from build123d import *

# Parameters (mm, degrees)
F0_R     = 8
F0_W     = 6.01
F0_H     = 18.1
F1_DEPTH = 6


with BuildPart() as f1:
    # F0 (on Front) → F1 (new body)
    with BuildSketch(Plane.XZ):
        Polygon((133.745999, -172.696896), (-31.254001, -172.696896), (-31.254001, -207.736896), (-25.244001, -207.736896), (-25.244001, -225.836896), (-31.254001, -225.836896), (-31.254001, -275.836896), (-25.244001, -275.836896), (-25.244001, -293.936896), (-31.254001, -293.936896), (-31.254001, -316.696896), (26.745999, -316.696896), (26.745999, -310.686896), (44.845999, -310.686896), (44.845999, -316.696896), (88.745999, -316.696896), (88.745999, -310.686896), (106.845999, -310.686896), (106.845999, -316.696896), (730.645999, -316.696896), (730.645999, -310.686896), (748.745999, -310.686896), (748.745999, -316.696896), (792.645999, -316.696896), (792.645999, -310.686896), (810.745999, -310.686896), (810.745999, -316.696896), (862.745999, -316.696896), (862.745999, -293.926896), (868.545999, -293.926896), (868.545999, -291.926896), (865.745999, -289.926896), (865.745999, -279.926896), (868.545999, -277.926896), (868.545999, -275.926896), (862.745999, -275.926896), (862.745999, -225.906896), (868.545999, -225.906896), (868.545999, -223.906896), (865.745999, -221.906896), (865.745999, -211.906896), (868.545999, -209.906896), (868.545999, -207.906896), (862.745999, -207.906896), (862.745999, -172.696896), (691.745999, -172.696896), (691.745999, -166.896896), (689.745999, -166.896896), (687.745999, -169.696896), (677.745999, -169.696896), (675.745999, -166.896896), (673.745999, -166.896896), (673.745999, -172.696896), (511.745999, -172.696896), (511.745999, -166.896896), (509.745999, -166.896896), (507.745999, -169.696896), (497.745999, -169.696896), (495.745999, -166.896896), (493.745999, -166.896896), (493.745999, -172.696896), (331.745999, -172.696896), (331.745999, -166.896896), (329.745999, -166.896896), (327.745999, -169.696896), (317.745999, -169.696896), (315.745999, -166.896896), (313.745999, -166.896896), (313.745999, -172.696896), (151.745999, -172.696896), (151.745999, -166.736896), (149.745999, -166.736896), (147.745999, -169.696896), (137.745999, -169.696896), (135.745999, -166.736896), (133.745999, -166.736896), align=None)
        with Locations((-6.254001, -291.696896)):
            Circle(F0_R, mode=Mode.SUBTRACT)
        with Locations((44.373021, -291.696896)):
            Circle(F0_R, mode=Mode.SUBTRACT)
        with Locations((94.373021, -291.696896)):
            Circle(F0_R, mode=Mode.SUBTRACT)
        with Locations((144.373021, -291.696896)):
            Circle(F0_R, mode=Mode.SUBTRACT)
        with Locations((161.750999, -284.886896)):
            Rectangle(F0_W, F0_H, mode=Mode.SUBTRACT)
        with Locations((194.373021, -291.696896)):
            Circle(F0_R, mode=Mode.SUBTRACT)
        with Locations((244.373021, -291.696896)):
            Circle(F0_R, mode=Mode.SUBTRACT)
        with Locations((294.373021, -291.696896)):
            Circle(F0_R, mode=Mode.SUBTRACT)
        with Locations((344.373021, -291.696896)):
            Circle(F0_R, mode=Mode.SUBTRACT)
        with Locations((394.373021, -291.696896)):
            Circle(F0_R, mode=Mode.SUBTRACT)
        with Locations((326.950999, -284.886896)):
            Rectangle(F0_W, F0_H, mode=Mode.SUBTRACT)
        with Locations((444.373021, -291.696896)):
            Circle(F0_R, mode=Mode.SUBTRACT)
        with Locations((494.373021, -291.696896)):
            Circle(F0_R, mode=Mode.SUBTRACT)
        with Locations((510.540999, -284.886896)):
            Rectangle(F0_W, F0_H, mode=Mode.SUBTRACT)
        with Locations((544.373021, -291.696896)):
            Circle(F0_R, mode=Mode.SUBTRACT)
        with Locations((594.373021, -291.696896)):
            Circle(F0_R, mode=Mode.SUBTRACT)
        with Locations((644.373021, -291.696896)):
            Circle(F0_R, mode=Mode.SUBTRACT)
        with Locations((694.373021, -291.696896)):
            Circle(F0_R, mode=Mode.SUBTRACT)
        with Locations((744.373021, -291.696896)):
            Circle(F0_R, mode=Mode.SUBTRACT)
        with Locations((675.740999, -284.886896)):
            Rectangle(F0_W, F0_H, mode=Mode.SUBTRACT)
        with Locations((794.373021, -291.696896)):
            Circle(F0_R, mode=Mode.SUBTRACT)
        with Locations((844.373021, -291.696896)):
            Circle(F0_R, mode=Mode.SUBTRACT)
        with Locations((-6.254001, -241.696896)):
            Circle(F0_R, mode=Mode.SUBTRACT)
        with Locations((44.373021, -241.696896)):
            Circle(F0_R, mode=Mode.SUBTRACT)
        with Locations((94.373021, -241.696896)):
            Circle(F0_R, mode=Mode.SUBTRACT)
        with Locations((144.373021, -241.696896)):
            Circle(F0_R, mode=Mode.SUBTRACT)
        with Locations((161.750999, -216.946896)):
            Rectangle(F0_W, F0_H, mode=Mode.SUBTRACT)
        with Locations((194.373021, -241.696896)):
            Circle(F0_R, mode=Mode.SUBTRACT)
        with Locations((244.373021, -241.696896)):
            Circle(F0_R, mode=Mode.SUBTRACT)
        with Locations((294.373021, -241.696896)):
            Circle(F0_R, mode=Mode.SUBTRACT)
        with Locations((344.373021, -241.696896)):
            Circle(F0_R, mode=Mode.SUBTRACT)
        with Locations((394.373021, -241.696896)):
            Circle(F0_R, mode=Mode.SUBTRACT)
        with Locations((326.950999, -216.946896)):
            Rectangle(F0_W, F0_H, mode=Mode.SUBTRACT)
        with Locations((-6.254001, -191.696896)):
            Circle(F0_R, mode=Mode.SUBTRACT)
        with Locations((44.373021, -191.696896)):
            Circle(F0_R, mode=Mode.SUBTRACT)
        with Locations((94.373021, -191.696896)):
            Circle(F0_R, mode=Mode.SUBTRACT)
        with Locations((144.373021, -191.696896)):
            Circle(F0_R, mode=Mode.SUBTRACT)
        with Locations((194.373021, -191.696896)):
            Circle(F0_R, mode=Mode.SUBTRACT)
        with Locations((244.373021, -191.696896)):
            Circle(F0_R, mode=Mode.SUBTRACT)
        with Locations((294.373021, -191.696896)):
            Circle(F0_R, mode=Mode.SUBTRACT)
        with Locations((344.373021, -191.696896)):
            Circle(F0_R, mode=Mode.SUBTRACT)
        with Locations((394.373021, -191.696896)):
            Circle(F0_R, mode=Mode.SUBTRACT)
        with Locations((444.373021, -241.696896)):
            Circle(F0_R, mode=Mode.SUBTRACT)
        with Locations((494.373021, -241.696896)):
            Circle(F0_R, mode=Mode.SUBTRACT)
        with Locations((544.373021, -241.696896)):
            Circle(F0_R, mode=Mode.SUBTRACT)
        with Locations((594.373021, -241.696896)):
            Circle(F0_R, mode=Mode.SUBTRACT)
        with Locations((510.540999, -216.946896)):
            Rectangle(F0_W, F0_H, mode=Mode.SUBTRACT)
        with Locations((644.373021, -241.696896)):
            Circle(F0_R, mode=Mode.SUBTRACT)
        with Locations((694.373021, -241.696896)):
            Circle(F0_R, mode=Mode.SUBTRACT)
        with Locations((744.373021, -241.696896)):
            Circle(F0_R, mode=Mode.SUBTRACT)
        with Locations((794.373021, -241.696896)):
            Circle(F0_R, mode=Mode.SUBTRACT)
        with Locations((844.373021, -241.696896)):
            Circle(F0_R, mode=Mode.SUBTRACT)
        with Locations((675.740999, -216.946896)):
            Rectangle(F0_W, F0_H, mode=Mode.SUBTRACT)
        with Locations((444.373021, -191.696896)):
            Circle(F0_R, mode=Mode.SUBTRACT)
        with Locations((494.373021, -191.696896)):
            Circle(F0_R, mode=Mode.SUBTRACT)
        with Locations((544.373021, -191.696896)):
            Circle(F0_R, mode=Mode.SUBTRACT)
        with Locations((594.373021, -191.696896)):
            Circle(F0_R, mode=Mode.SUBTRACT)
        with Locations((644.373021, -191.696896)):
            Circle(F0_R, mode=Mode.SUBTRACT)
        with Locations((694.373021, -191.696896)):
            Circle(F0_R, mode=Mode.SUBTRACT)
        with Locations((744.373021, -191.696896)):
            Circle(F0_R, mode=Mode.SUBTRACT)
        with Locations((794.373021, -191.696896)):
            Circle(F0_R, mode=Mode.SUBTRACT)
        with Locations((844.373021, -191.696896)):
            Circle(F0_R, mode=Mode.SUBTRACT)
    extrude(amount=F1_DEPTH)


solid = f1.part
Could you check a few things on this model? Use its own coordinates, in mm. Give positions to 0.01 mm unless a question says otherwise; leave off trailing zeros. Order: outer loops, then holes, each group sorted by start corner. A loop starts at its lowest first (then second) coordinate and runs counter-clockwise, first axis right, second up. Notation, with made-up numbers: (89.25, 60) - (132.25, 60) arc R16 cw to (132.25, 69) - close; hole circle Ø2 at (60, 9.25). An arc over 180 degrees is marked (long way). Return JSON: item names as keys, results as strings. Group by question number.
Q1. Suppose I cut it at B-B, the plane y = -2.85. State how many separate pieces and enclosed holes the cut face has, and give its area (3 significant figures).
Q2. Suppose I cut it at A-A, the plane x = 66. Please give me the cut outline in (y, z).
Q3. Will these pins go through, and if not, where does the flat tip stop? pin 1 Ø18.5 at (x, z) = (94.37, -291.7) entering from -Y; pin 2 Ø1.8 at (y, z) = (-3, -314) entering from +X; pin 3 Ø3 at (x, y) = (328, -2) entering from +Z; pin 4 Ø1.6 at (x, y) = (330.5, -3.5) entering from +Z.
Q4. Thinking about a two-plate mould opening in Z: for faces 1 (the face through (412, -6, -241)), 2 (the face through (48.065, -2.958, -248.794)), which applies, pulls with the +Z half, pulls with the -Z half, needs draft (parallel to the pull), parting line crosses it, or undercut?
Q5. Please list where these lines run through material, in increasing order: line 1 along X through (y, z) = (-5.15, -209.5); line 2 along X through (y, z) = (-4.85, -216); line 3 along Z through (x, y) = (341.5, -1.85). Write a range as [from, to].
Resolved:
{
 "1": {"separate pieces": "1", "enclosed holes": "62", "area": "117,000 mm2"},
 "2": {"outline": "(-6, -316.7) - (0, -316.7) - (0, -172.7) - (-6, -172.7) - close"},
 "3": {"pin 1": "stops at y = -6", "pin 2": "stops at x = 862.75", "pin 3": "stops at z = -167.24", "pin 4": "stops at z = -166.9"},
 "4": {"face 1": "needs draft", "face 2": "undercut"},
 "5": {"line 1": "x = [-25.24, 158.75], [164.76, 323.95], [329.96, 507.54], [513.55, 672.74], [678.75, 868.55]", "line 2": "x = [-25.24, 158.75], [164.76, 323.95], [329.96, 507.54], [513.55, 672.74], [678.75, 865.75]", "line 3": "z = [-316.7, -299.16], [-284.23, -249.16], [-234.23, -199.16], [-184.23, -172.7]"}
}
